Model file for the job. Use its own axes, mm. Face numbers are marked on the shaded views. A direction names the side the tool comes from. Give positions to 0.01 mm unless a question says otherwise; leave off trailing zeros. Write each loop counter-clockwise with the first axis right and the second up, starting at its lowest first coordinate (ties: lowest second). Pieces come first, ordered by that corner, then holes. Notation, with made-up numbers: (86.25, 78) - (137.25, 78) arc R26 ccw to (137.25, 102) - close; hole circle Ø10 at (44, 31.5). An arc over 180 degrees is marked (long way). Use CSV: the item, a comma, the result in double quotes.
Autodesk Fusion 360 part; units mm, degrees
sketch "Sketch1" plane through (0, 0, 0) normal (0, 0, 1) x (1, 0, 0)
  line L0 (-26.0373, -33.6026) -> (-1.0373, -33.6026)
  line L1 (-1.0373, -33.6026) -> (-1.0373, 36.3974)
  line L2 (-1.0373, 36.3974) -> (-26.0373, 36.3974)
  line L3 (-26.0373, 36.3974) -> (-26.0373, -33.6026)
  dimension "d1" = 25
  dimension "d2" = 70
extrude "Extrude1" add sketch "Sketch1" along normal blind 3
extrude "Extrude2" add 1 faces at (-17.7039, 13.0641, 3) along direction (0, 0, 1) blind 5
sketch "Sketch2" plane through (0, 0, 8) normal (0, 0, 1) x (-1, 0, 0)
  line L0 (26.0373, -36.3974) -> (26.0373, 33.6026)
  line L1 (26.0373, 33.6026) -> (1.0373, 33.6026)
  line L2 (1.0373, 33.6026) -> (1.0373, -36.3974)
  line L3 (1.0373, -36.3974) -> (26.0373, -36.3974)
  line L4 (23.98, -34.1191) -> (3.337, -34.1191)
  line L5 (3.337, -34.1191) -> (3.337, 31.543)
  line L6 (3.337, 31.543) -> (23.98, 31.543)
  line L7 (23.98, 31.543) -> (23.98, -34.1191)
extrude "Extrude3" cut sketch "Sketch2" against normal blind 5 contours L4 L5 L6 L7
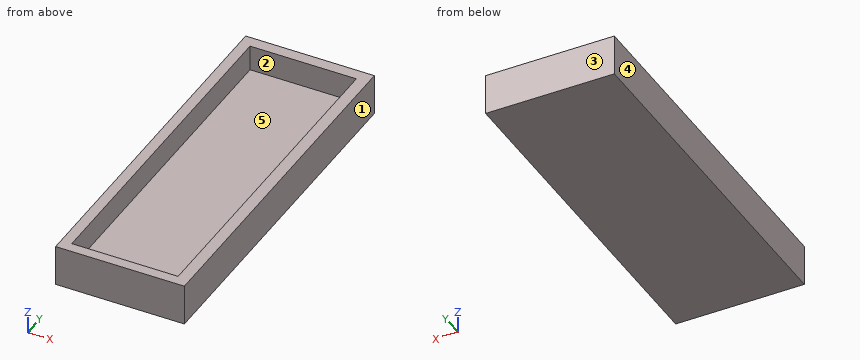
(1) Saw through at C-C, the plane x = -19. List the corners of the cut face in (y, z).
Checked values:
outline,"(-33.6, 0) - (36.4, 0) - (36.4, 8) - (34.12, 8) - (34.12, 3) - (-31.54, 3) - (-31.54, 8) - (-33.6, 8) - close"
(2) Pull direction X, two halves, no side cores. Call the marked faces 1, 2 and 3: released by +X, released by -X, zero draft, split by the parting line, or undercut.
Checked values:
face 1,"released by +X"
face 2,"undercut"
face 3,"zero draft"
(3) Flat gauge pin, fed straight in: P1, Ø1, axis at x = -10.5, y = 6, coming from the +Z side. Where does the tip first touch, or does it go through?
Checked values:
P1,"stops at z = 3"
(4) 3-axis set-ups, long thin cutter, end or side, ignore diameter. For the marked faces 4 and 5: which of +Z, -Z, +X, -X, +Y, -Y reach the whole face in a straight line?
Checked values:
face 4,"+Z, -Z, -X, +Y, -Y"
face 5,"+Z"
(5) Saw through at B-B, the plane y = -3. List the corners of the cut face in (x, z), then the cut area to 3 significant figures.
Checked values:
outline,"(-26.04, 0) - (-1.04, 0) - (-1.04, 8) - (-3.34, 8) - (-3.34, 3) - (-23.98, 3) - (-23.98, 8) - (-26.04, 8) - close"
area,"96.8 mm^2"
(6) Saw through at A-A, the plane z = 6.5. List the corners of the cut face in (x, y).
Checked values:
outline,"(-26.04, -33.6) - (-1.04, -33.6) - (-1.04, 36.4) - (-26.04, 36.4) - close; hole (-23.98, -31.54) - (-3.34, -31.54) - (-3.34, 34.12) - (-23.98, 34.12) - close"
(7) Wall check: probe 1 along X at (y, z) = (31, 3.75); probe 2 along Y at (x, z) = (-6.75, 3.25); probe 3 along Z at (x, y) = (-5.5, 16.5). Give the ranges that are in metal, low to high. Write a range as [from, to].
Checked values:
probe 1,"x = [-26.04, -23.98], [-3.34, -1.04]"
probe 2,"y = [-33.6, -31.54], [34.12, 36.4]"
probe 3,"z = [0, 3]"
